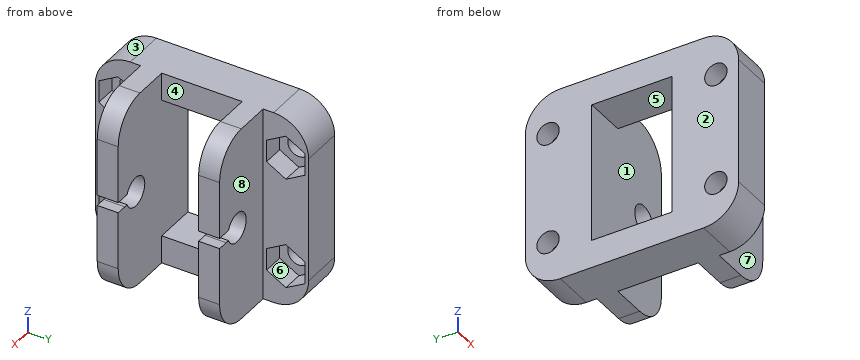
Solid Edge part; units mm, degrees
sketch "Sketch1" plane through (0, 0, 0) normal (1, 0, 0) x (0, 1, 0)
  circle A0 centre (32.3514, 23.2437) radius 1.6
  circle A1 centre (56.3514, 23.2437) radius 1.6
  circle A2 centre (56.3514, 39.2437) radius 1.6
  line L0 (59.6014, 17.2437) -> (59.6014, 45.2437)
  line L1 (29.1014, 45.2437) -> (59.6014, 45.2437)
  line L2 (29.1014, 45.2437) -> (29.1014, 17.2437)
  line L3 (59.6014, 17.2437) -> (29.1014, 17.2437)
  line L4 (38.6014, 21.2437) -> (50.1014, 21.2437)
  line L5 (50.1014, 21.2437) -> (50.1014, 41.2437)
  line L6 (50.1014, 41.2437) -> (38.6014, 41.2437)
  line L7 (38.6014, 41.2437) -> (38.6014, 21.2437)
  circle A3 centre (32.3514, 39.2437) radius 1.6
extrude "Protrusion1" add sketch "Sketch1" along normal blind 6
sketch "Sketch2" plane through (6, 44.3514, 31.2437) normal (1, 0, 0) x (0, 1, 0)
  line L0 (-5.75, 14) -> (-8.75, 14)
  line L1 (-8.75, 14) -> (-8.75, -14)
  line L2 (-8.75, -14) -> (-5.75, -14)
  line L3 (-5.75, 14) -> (-5.75, -14)
  line L4 (5.75, 14) -> (8.75, 14)
  line L5 (8.75, 14) -> (8.75, -14)
  line L6 (8.75, -14) -> (5.75, -14)
  line L7 (5.75, -14) -> (5.75, 14)
  dimension "D1" = 5.75
  dimension "D2" = 8.75
  dimension "D3" = 8.75
extrude "ExtrudedProtrusion_2" add sketch "Sketch2" along normal blind 10
sketch "Sketch3" plane through (6, 44.3514, 31.2437) normal (1, 0, 0) x (0, 1, 0)
  line L0 (-9.25, 9.5877) -> (-12, 11.1754)
  line L1 (-12, 11.1754) -> (-14.75, 9.5877)
  line L2 (-14.75, 9.5877) -> (-14.75, 6.4123)
  line L3 (-14.75, 6.4123) -> (-12, 4.8246)
  line L4 (-12, 4.8246) -> (-9.25, 6.4123)
  line L5 (-9.25, 6.4123) -> (-9.25, 9.5877)
  line L6 (-9.25, -6.4123) -> (-12, -4.8246)
  line L7 (-12, -4.8246) -> (-14.75, -6.4123)
  line L8 (-14.75, -6.4123) -> (-14.75, -9.5877)
  line L9 (-14.75, -9.5877) -> (-12, -11.1754)
  line L10 (-12, -11.1754) -> (-9.25, -9.5877)
  line L11 (-9.25, -9.5877) -> (-9.25, -6.4123)
  line L12 (14.75, 9.5877) -> (12, 11.1754)
  line L13 (12, 11.1754) -> (9.25, 9.5877)
  line L14 (9.25, 9.5877) -> (9.25, 6.4123)
  line L15 (9.25, 6.4123) -> (12, 4.8246)
  line L16 (12, 4.8246) -> (14.75, 6.4123)
  line L17 (14.75, 6.4123) -> (14.75, 9.5877)
  line L18 (14.75, -6.4123) -> (12, -4.8246)
  line L19 (12, -4.8246) -> (9.25, -6.4123)
  line L20 (9.25, -6.4123) -> (9.25, -9.5877)
  line L21 (9.25, -9.5877) -> (12, -11.1754)
  line L22 (12, -11.1754) -> (14.75, -9.5877)
  line L23 (14.75, -9.5877) -> (14.75, -6.4123)
extrude "ExtrudedCutout_1" cut sketch "Sketch3" against normal blind 3
sketch "Sketch4" plane through (11, 35.6014, 31.2437) normal (0, -1, 0) x (1, 0, 0)
  line L0 (3.4895, 0.75) -> (7.5, 0.75)
  line L1 (7.5, 0.75) -> (7.5, -0.75)
  line L2 (7.5, -0.75) -> (3.4895, -0.75)
  line L3 (3.4895, -0.75) -> (2.9615, -0.75)
  line L4 (3.4895, 0.75) -> (2.9615, 0.75)
  arc A0 (2.9615, 0.75) -> (2.9615, -0.75) centre (1, 0) ccw
extrude "ExtrudedCutout_2" cut sketch "Sketch4" against normal blind 20
fillet "Round_1" radius 5 8 edges at (16, 37.1014, 45.2437) (16, 51.6014, 45.2437) (16, 37.1014, 17.2437) (16, 51.6014, 17.2437) (3, 29.1014, 17.2437) (3, 29.1014, 45.2437) (3, 59.6014, 45.2437) (3, 59.6014, 17.2437)
Can you work these out from the model? Positions are in its coordinate system, mm. Face numbers are marked on the shaded views. A direction names the side the tool comes from. Round coordinates to 2 decimals unless told otherwise and drop trailing zeros. Loops run counter-clockwise (first coordinate to the right, second up) from the corner with the lowest first, then second, coordinate; pieces in that order, holes last. Notation, with made-up numbers: (-16, -32) - (36, -32) arc R34 ccw to (36, 0) - close; hole circle Ø11 at (52.25, 28.5). An arc over 180 degrees is marked (long way). Answer in a Markdown table with one row per item. Add a question column.
Q1. I want a section at D-D on x = 12. List the corners of the cut face in (y, z) for me.
Q2. I need wall thicknesses on L1, parallel to Y at x = 5.25, z = 39; L2, parallel to Y at x = 9.5, z = 30; L3, parallel to Z at x = 5.25, y = 47. Which ranges of each line are inside material? Lowest first, please.
Q3. Which directions (+Z, -Z, +X, -X, +Y, -Y) give clear straight access to the entire face, cutting with the end or side of a thin tool? Please do the marked faces 4, 5, 6, 7 and 8.
Q4. I want a section at B-B on x = 7.75. List the corners of the cut face in (y, z) for me.
Q5. For pin 1 Ø4 at (x, z) = (12, 32) entering from +Y; pin 2 Ø1.2 at (x, y) = (15.5, 52) entering from -Z; pin 3 Ø1.2 at (x, y) = (15, 51) entering from +Z, each with a flat end and sliding along its axis, tell me the tip position at first contact or that it passes through.
Q6. I want a section at A-A on z = 34.75. List the corners of the cut face in (x, y) for me, and give its area (3 significant figures).
Q7. I want a section at C-C on z = 38.25. List the corners of the cut face in (x, y) for me.
Q8. We'd pull the mould along Z, two halves only. Please class the marked faces 1, 2 and 3: pulls with the +Z half, pulls with the -Z half, needs draft (parallel to the pull), parting line crosses it, or undercut.
A:
| question | item | result |
|---|---|---|
| 1 | outline | (35.6, 17.34) - (38.6, 17.34) - (38.6, 29.14) - (35.6, 29.14) - close; (35.6, 33.34) - (38.6, 33.34) - (38.6, 45.14) - (35.6, 45.14) - close; (50.1, 17.34) - (53.1, 17.34) - (53.1, 29.14) - (50.1, 29.14) - close; (50.1, 33.34) - (53.1, 33.34) - (53.1, 45.14) - (50.1, 45.14) - close |
| 2 | L1 | 29.1 to 29.6, 35.1 to 38.6, 50.1 to 53.6, 59.1 to 59.6 |
| 2 | L2 | 35.6 to 38.6, 50.1 to 53.1 |
| 2 | L3 | 17.24 to 21.24, 41.24 to 45.24 |
| 3 | face 4 | +Z, -Z, +X |
| 3 | face 5 | +X, -X |
| 3 | face 6 | +X |
| 3 | face 7 | +Z, -Z, +X, -Y |
| 3 | face 8 | +Z, -Z, +X, +Y |
| 4 | outline | (35.6, 17.24) - (38.6, 17.24) - (38.6, 45.24) - (35.6, 45.24) - close; (50.1, 17.24) - (53.1, 17.24) - (53.1, 45.24) - (50.1, 45.24) - close |
| 5 | pin 1 | y = 53.1 |
| 5 | pin 2 | z = 19.11 |
| 5 | pin 3 | z = 43.91 |
| 6 | outline | (0, 29.1) - (6, 29.1) - (6, 35.6) - (16, 35.6) - (16, 38.6) - (0, 38.6) - close; (0, 50.1) - (16, 50.1) - (16, 53.1) - (6, 53.1) - (6, 59.6) - (0, 59.6) - close |
| 6 | area | 174 mm^2 |
| 7 | outline | (0, 29.1) - (6, 29.1) - (6, 29.6) - (3, 29.6) - (3, 31.1) - (0, 31.1) - close; (0, 33.61) - (3, 33.61) - (3, 35.1) - (6, 35.1) - (6, 35.6) - (16, 35.6) - (16, 38.6) - (0, 38.6) - close; (0, 50.1) - (16, 50.1) - (16, 53.1) - (6, 53.1) - (6, 53.6) - (3, 53.6) - (3, 55.1) - (0, 55.1) - close; (0, 57.61) - (3, 57.61) - (3, 59.1) - (6, 59.1) - (6, 59.6) - (0, 59.6) - close |
| 8 | face 1 | undercut |
| 8 | face 2 | needs draft |
| 8 | face 3 | pulls with the +Z half |
